The figure shows three views and two pictorial views of one solid part (mm, origin at its lowest corner). Answer the questions. Coordinates: 2 decimals unless noted, no trailing zeros. Order: outer loops, then holes, each group sorted by start corner. A loop starts at its lowest first (then second) coordinate and runs counter-clockwise, first axis right, second up.
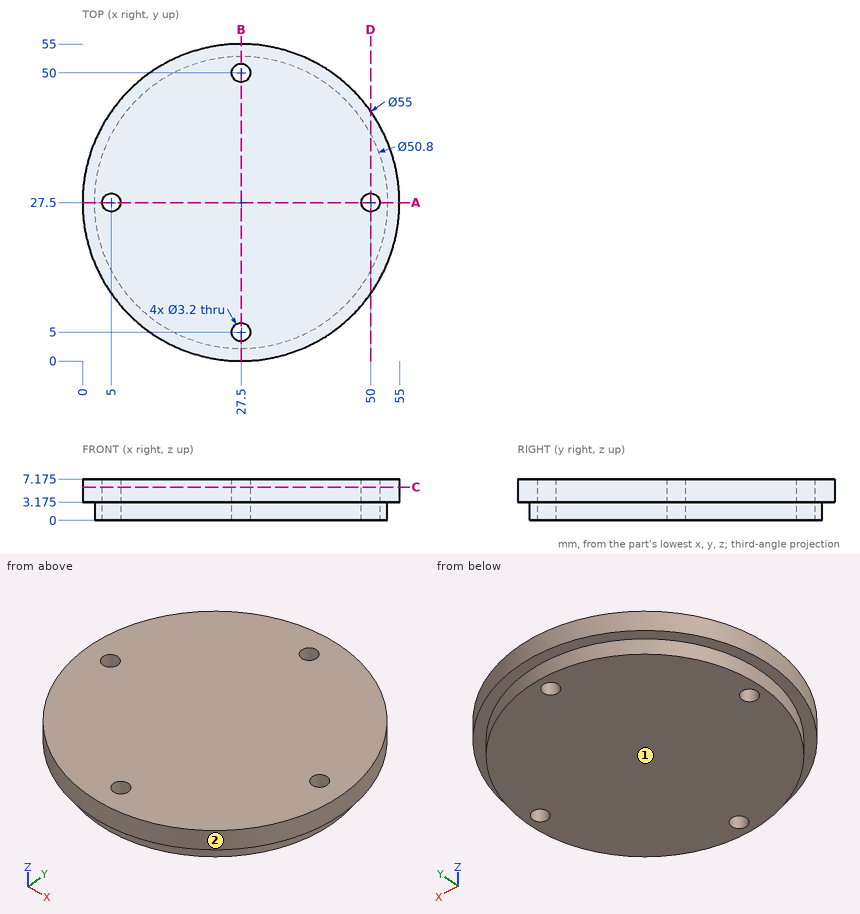
Q1. The part is cut by section C-C, the plane z = 5.75. Determine the outline of the cut face in (x, y), then the cut area to 3 significant figures.
Q2. The part is cut by section D-D, the plane x = 50. Determine the outline of the cut face in (y, z) (3 decimals).
Q3. The part is cut by section A-A, the plane y = 27.5. Determine the outline of the cut face in (x, z) (3 decimals), then the cut area to 3 significant figures.
Q4. Each of these flat-tipped pins is pushed along its axis until it touches: P1, Ø1, axis at x = 32, z = 3.5, coming from the +Y side; P2, Ø2, axis at x = 48.5, z = 5, coming from the -Y side; P3, Ø4, axis at x = 15.5, z = 1.5, coming from the +Y side; P4, Ø1.9, axis at x = 50, y = 27.5, coming from the -Z side. Where does it stop, or does it pass through?
Q5. Determine the mould class of the marked faces 1 and 2 for opening direction X: +X half, -X half, draft (parallel to the pull), parting line (faces both ways), or undercut.
Q6. Straight lines are drawn through the part: L1, parallel to Y at x = 50, z = 6; L2, parallel to Y at x = 5, z = 2; L3, parallel to X at y = 43.5, z = 1. For each, find the intervals that lie inside material, in ascending order.
Computed values:
1. outline: circle Ø55 at (27.5, 27.5); hole circle Ø3.2 at (5, 27.5); hole circle Ø3.2 at (27.5, 5); hole circle Ø3.2 at (27.5, 50); hole circle Ø3.2 at (50, 27.5)
1. area: 2,340 mm2
2. outline: (11.689, 3.175) - (15.714, 3.175) - (15.714, 0) - (25.9, 0) - (25.9, 7.175) - (11.689, 7.175) - close; (29.1, 0) - (39.286, 0) - (39.286, 3.175) - (43.311, 3.175) - (43.311, 7.175) - (29.1, 7.175) - close
3. outline: (0, 3.175) - (2.1, 3.175) - (2.1, 0) - (3.4, 0) - (3.4, 7.175) - (0, 7.175) - close; (6.6, 0) - (48.4, 0) - (48.4, 7.175) - (6.6, 7.175) - close; (51.6, 0) - (52.9, 0) - (52.9, 3.175) - (55, 3.175) - (55, 7.175) - (51.6, 7.175) - close
3. area: 335 mm2
4. P1: stops at y = 54.71
4. P2: stops at y = 8.63
4. P3: stops at y = 52.74
4. P4: passes through
5. face 1: draft
5. face 2: parting line
6. L1: y = 11.69 to 25.9, 29.1 to 43.31
6. L2: y = 15.71 to 25.9, 29.1 to 39.29
6. L3: x = 7.77 to 47.23
